```python
from build123d import *

# Parameters (mm, degrees)
SKETCH2_R               = 6
CUT_EXTRUDE1_DEPTH      = 405.418100485
CUT_EXTRUDE3_DEPTH      = 301.562805417
CUT_EXTRUDE3_DEPTH_BACK = 301.562805417
SKETCH3_R               = 4
FILLET1_R               = 1


with BuildPart() as part:
    # Sketch1 → Revolve1 (revolve)
    with BuildSketch(Plane(origin=(0, 0, 0), x_dir=(0, 0, -1), z_dir=(1, 0, 0))):
        Polygon((0, 0), (0, 300), (10, 300), (10, 0), (13, 0), (13, -4), (8, -4), (8, -104), (0, -104), align=None)
    revolve(axis=Axis((0, 0, 0), (0, 1, 0)))

    # Sketch2 → Cut-Extrude1 (cut, through all)
    with BuildSketch(Plane(origin=(0, 300, 0), x_dir=(1, 0, 0), z_dir=(0, 1, 0))):
        with Locations(Location((0, 0, 0), (0, 0, 270))):
            Circle(SKETCH2_R)
    extrude(amount=-CUT_EXTRUDE1_DEPTH, mode=Mode.SUBTRACT)

    # Sketch3 → Cut-Extrude3 (cut, two sides: drawn at the far end of the back side and taken through both)
    with BuildSketch(Plane(origin=(0, 0, 0), x_dir=(0, 0, -1), z_dir=(1, 0, 0)).offset(-CUT_EXTRUDE3_DEPTH_BACK)):
        with Locations((0, -14)):
            Circle(SKETCH3_R)
        with Locations((0, -69)):
            Circle(SKETCH3_R)
        with Locations((0, -89)):
            Circle(SKETCH3_R)
    extrude(amount=CUT_EXTRUDE3_DEPTH + CUT_EXTRUDE3_DEPTH_BACK, mode=Mode.SUBTRACT)

    # Fillet1
    fillet1_edges = [part.edges().sort_by_distance(p)[0] for p in [
        (0, -4, 13),
        (0, 0, 13),
    ]]
    fillet(fillet1_edges, radius=FILLET1_R)


solid = part.part
```
CAD build for the part. Positions are in the model's coordinates, mm. A direction names the side the tool comes from. Round coordinates to 2 decimals unless told otherwise and drop trailing zeros. Write each loop counter-clockwise with the first axis right and the second up, starting at its lowest first coordinate (ties: lowest second). Pieces come first, ordered by that corner, then holes. Notation, with made-up numbers: (63, 2.25) -> (101, 2.25) arc R27 cw to (101, 25.25) -> close; hole circle Ø8 at (67.25, 11.5). An arc over 180 degrees is marked (long way). Answer in a Markdown table with one row per item. Add a question column.
Item 1: Which spindle directions (+Z, -Z, +X, -X, +Y, -Y) get a long thin tool onto all of the face, cutting with end or side? Do faces 5 (the face through (-9, 0, -5)), 6 (the face through (-6.261, -90.532, -3.695)), 7 (the face through (8, -4, -2)). Say none if no direction does.
Item 2: Saw through at B-B, the plane y = -14. Write the cut outline in (x, z), then the cut area to 3 significant figures.
Item 3: Mould opens along Y. For faces 1 (the face through (-6.261, -67.799, -3.815)), 2 (the face through (9.76, 147.9, 2.17)), 3 (the face through (6.212, -87.799, -3.815)), 4 (the face through (-6, -104, 2)) say: pulls with the +Y half, pulls with the -Y half, needs draft (parallel to the pull), parting line crosses it, or undercut.
Item 4: Saw through at C-C, the plane z = 0. Count the separate pieces of the cut face and the enclosed holes in it, then the cut area to 3 significant figures.
Item 5: Saw through at D-D, the plane y = 89. Write the cut outline in (x, z).
Item 6: Drill centre lines: line 1 (Y direction, x = 7, z = 0.75); line 2 (Y direction, x = 7.25, z = 0); line 3 (X direction, y = 160, z = -0.25). Where is each one in solid material? Low to high. Write a range as from..to.
Item 7: Saw through at A-A, the plane x = 0. Write the cut outline in (y, z), then the cut area to 3 significant figures.
Item 8: Drop flat-ended pins along their axis: pin 1 Ø1.5 at (x, y) = (0.5, 259.5) entering from -Z; pin 2 Ø4 at (y, z) = (78.5, 8.5) entering from +X; pin 3 Ø13 at (y, z) = (-69, 0) entering from +X; pin 4 Ø6.5 at (y, z) = (-14, 0) entering from +X. Give the stop position or say it passes through.
Findings below:
| question | item | result |
|---|---|---|
| 1 | face 5 | +Y |
| 1 | face 6 | +X, -X |
| 1 | face 7 | -Y |
| 2 | outline | (-6.93, -4) arc R8 ccw to (6.93, -4) -> (4.47, -4) arc R6 cw to (-4.47, -4) -> close; (-6.93, 4) -> (-4.47, 4) arc R6 cw to (4.47, 4) -> (6.93, 4) arc R8 ccw to start |
| 2 | area | 53.8 mm^2 |
| 3 | face 1 | undercut |
| 3 | face 2 | needs draft |
| 3 | face 3 | undercut |
| 3 | face 4 | pulls with the -Y half |
| 4 | separate pieces | 8 |
| 4 | enclosed holes | 0 |
| 4 | area | 2,760 mm^2 |
| 5 | outline | circle Ø20 at (0, 0); hole circle Ø12 at (0, 0) |
| 6 | line 1 | y = -104..-92.93, -85.07..-72.93, -65.07..-17.93, -10.07..300 |
| 6 | line 2 | y = -104..-93, -85..-73, -65..-18, -10..300 |
| 6 | line 3 | x = -10..-5.99, 5.99..10 |
| 7 | outline | (-104, -8) -> (-4, -8) -> (-4, -12) arc R1 ccw to (-3, -13) -> (-1, -13) arc R1 ccw to (0, -12) -> (0, -10) -> (300, -10) -> (300, -6) -> (-104, -6) -> close; (-104, 6) -> (300, 6) -> (300, 10) -> (0, 10) -> (0, 12) arc R1 ccw to (-1, 13) -> (-3, 13) arc R1 ccw to (-4, 12) -> (-4, 8) -> (-104, 8) -> close |
| 7 | area | 2,860 mm^2 |
| 8 | pin 1 | stops at z = -10 |
| 8 | pin 2 | stops at x = 7.6 |
| 8 | pin 3 | stops at x = 8 |
| 8 | pin 4 | passes through |
